Design review of the part built by this model. Coordinates are the model's own, in mm. Face numbers are marked on the shaded views. Give positions to 0.01 mm unless a question says otherwise; leave off trailing zeros. Loops run counter-clockwise (first coordinate to the right, second up) from the corner with the lowest first, then second, coordinate; pieces in that order, holes last. Notation, with made-up numbers: (39, 50.5) -> (76, 50.5) arc R36 cw to (76, 89.5) -> close; hole circle Ø2 at (-23, -38.5). An arc over 180 degrees is marked (long way). Use CSV: the item, a comma, the result in double quotes. Start each with the question number.
Item 1: We need section A-A (z = 0). State the section outline as (x, y) points.
Item 2: We need section B-B (x = 0). State the section outline as (y, z) points.
Item 3: We need section C-C (y = 2.5). State the section outline as (x, z) points, plus the area to 3 significant figures.
Item 4: Wall thickness on line 1 along Y through (x, z) = (-16, 0); line 2 along X through (y, z) = (4, -9.5); line 3 along Z through (x, y) = (-7.5, 6.75): over which ranges is each line inside the solid? List them lowest first. Write a range as from..to.
Item 5: Clearance check with flat-ended pins moving along their axes: pin 1 (4 mm diameter, centred on x = -5, y = 4.5, fed in from +Z); pin 2 (1 mm diameter, centred on x = -12.5, y = 2, fed in from -Z); pin 3 (2 mm diameter, centred on y = 1, z = 14, fed in from +X); pin 4 (13 mm diameter, centred on x = -0.5, z = 4.5, fed in from +Y) (3 decimals). State where each tip first meets the part, or that it passes through.
Item 6: The part is to be moulded in two halves that separate along X. For the marked faces 1, 2 and 3, say which applies: +X half, -X half, draft (parallel to the pull), parting line (faces both ways), or undercut.
Item 7: We need section D-D (x = 8). Count the separate pieces of the cut face and the enclosed holes in it, plus the area to 3 significant figures.
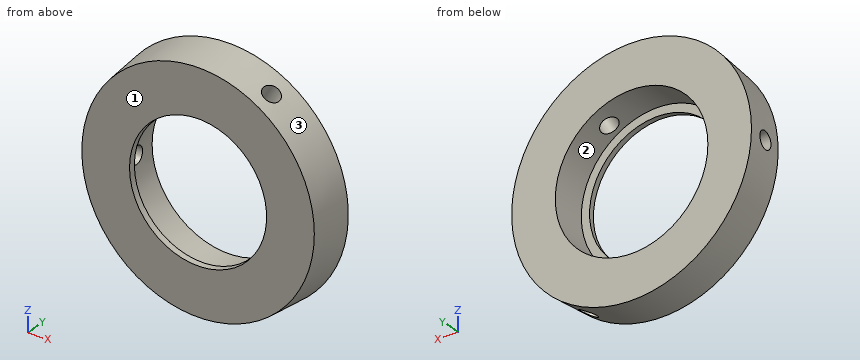
Autodesk Inventor part; units mm, degrees
ref_plane "YZ Plane" through (0, 0, 0) normal (1, 0, 0) x (0, 1, 0)
ref_plane "XZ Plane" through (0, 0, 0) normal (0, 1, 0) x (-1, 0, 0)
ref_plane "XY Plane" through (0, 0, 0) normal (0, 0, 1) x (1, 0, 0)
sketch "Skizze1" plane through (0, 0, 0) normal (0, 1, 0) x (-1, 0, 0)
  circle A0 centre (0, 0) radius 19.5
  line L0 (-8, 0) -> (8, 0) construction
  circle A1 centre (0, 0) radius 11.5
  dimension "d0" = 39
  dimension "d1" = 8
  dimension "d8" = 23
extrude "Extrusion1" add sketch "Skizze1" along normal blind 7 draft 5
sketch "Skizze2" plane through (0, 7, 0) normal (0, 1, 0) x (1, 0, 0)
  circle A0 centre (0, 0) radius 20.1124
  circle A1 centre (0, 0) radius 12.8
  dimension "d5" = 25.6
extrude "Extrusion2" cut sketch "Skizze2" against normal blind 6 contours A1
sketch "Skizze3" plane through (0, 0, 0) normal (1, 0, 0) x (0, 1, 0)
  line L0 (7, 20.1124) -> (7, -20.1124)
  line L1 (0, -19.5) -> (0, 19.5)
  circle A0 centre (3.3414, 0) radius 1.45
  point P0 (0, 0)
  dimension "d9" = 2.9
extrude "Extrusion3" cut sketch "Skizze3" against normal through all
pattern_circular "Runde Anordnung1" count 3 over 360 about axis through (0, 7, 0) along (0, -1, 0) of "Extrusion3"
properties part number "50_Filteradapter_Fluorescence_CCVTV_Berrybase_100mm"
Results found:
1,outline,"(-20.11, 7) -> (-19.92, 4.79) -> (-12.8, 4.79) -> (-12.8, 7) -> close; (-19.67, 1.89) -> (-19.5, 0) -> (-11.5, 0) -> (-11.41, 1) -> (-12.8, 1) -> (-12.8, 1.89) -> close; (11.41, 1) -> (11.5, 0) -> (19.5, 0) -> (20.11, 7) -> (12.8, 7) -> (12.8, 1) -> close"
2,outline,"(0, -19.5) -> (7, -20.11) -> (7, -12.8) -> (1, -12.8) -> (1, -11.41) -> (0, -11.5) -> close; (0, 11.5) -> (1, 11.41) -> (1, 12.8) -> (7, 12.8) -> (7, 20.11) -> (0, 19.5) -> close"
3,outline,"(-19.68, -1.18) arc R19.72 ccw to (8.82, -17.64) -> (5.35, -11.63) arc R12.8 cw to (-12.75, -1.18) -> close; (-19.68, 1.18) -> (-12.75, 1.18) arc R12.8 cw to (5.35, 11.63) -> (8.82, 17.64) arc R19.72 ccw to start; (7.4, -10.45) -> (10.86, -16.46) arc R19.72 ccw to (10.86, 16.46) -> (7.4, 10.45) arc R12.8 cw to start"
3,area,"658 mm²"
4,line 1,"0..1.89, 4.79..7"
4,line 2,"-17.43..-8.58, 8.58..17.43"
4,line 3,"-18.64..-10.37, 10.37..18.64"
5,pin 1,"z = 19.71"
5,pin 2,"z = -15.6"
5,pin 3,"x = 14.66"
5,pin 4,"through"
6,face 1,"draft"
6,face 2,"undercut"
6,face 3,"parting line"
7,separate pieces,"2"
7,enclosed holes,"2"
7,area,"90.9 mm²"
